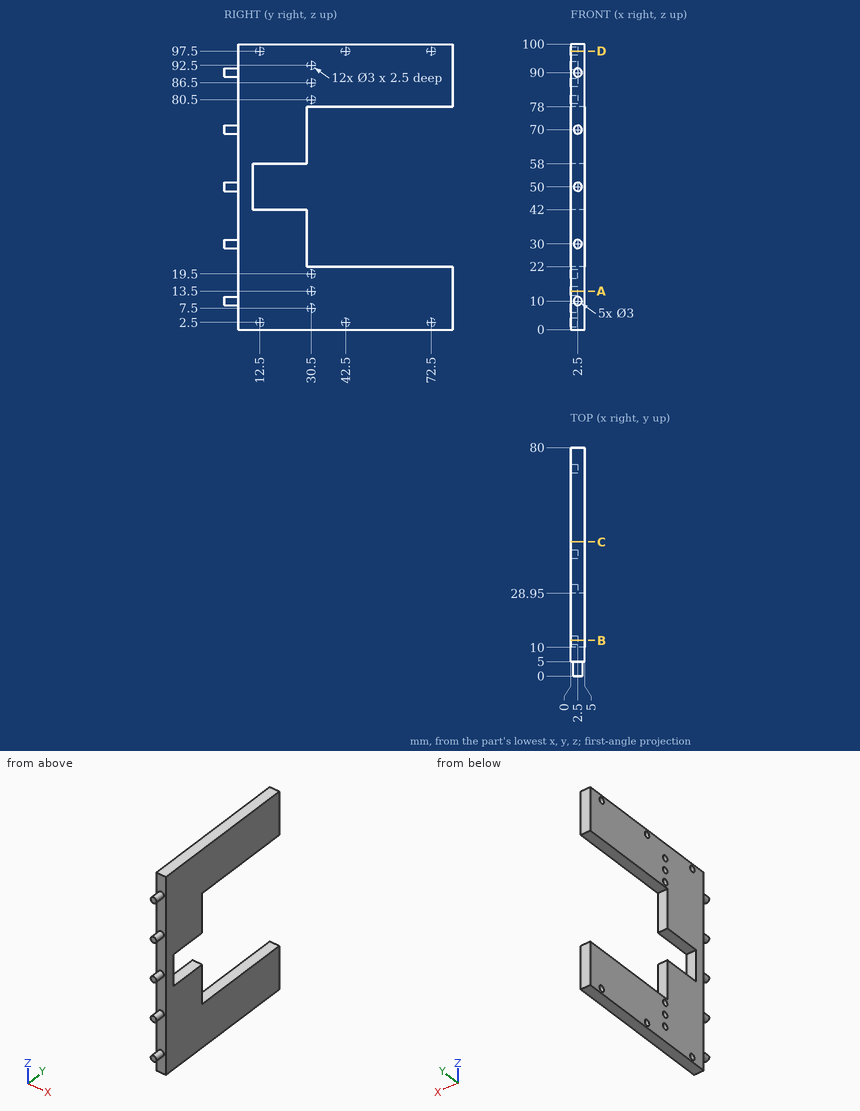
Geometry check sheet. Reference: drawing and pictorial views, mm from the part's lowest x, y, z. Coordinates: 2 decimals unless noted, no trailing zeros. Order: outer loops, then holes, each group sorted by start corner. A loop starts at its lowest first (then second) coordinate and runs counter-clockwise, first axis right, second up.
1. Scan lines: line 1 (Y direction, x = 1.1, z = 97.5); line 2 (Z direction, x = 2.4, y = 15); line 3 (Y direction, x = 0.6, z = 13.5). Record each from-to range of solid material in increasing order.
Results found:
line 1: y = 5 to 11, 14 to 41, 44 to 71, 74 to 80
line 2: z = 0 to 42, 58 to 100
line 3: y = 5 to 29, 32 to 80
2. Sectioned sample at A-A, the plane z = 13.5. Record the cut outline in (x, y).
Results found:
outline: (0, 5) - (5, 5) - (5, 80) - (0, 80) - (0, 32) - (2.5, 32) - (2.5, 29) - (0, 29) - close
3. Sectioned sample at D-D, the plane z = 97.5. Record the cut outline in (x, y).
Results found:
outline: (0, 5) - (5, 5) - (5, 80) - (0, 80) - (0, 74) - (2.5, 74) - (2.5, 71) - (0, 71) - (0, 44) - (2.5, 44) - (2.5, 41) - (0, 41) - (0, 14) - (2.5, 14) - (2.5, 11) - (0, 11) - close
4. Sectioned sample at C-C, the plane y = 47. Record the cut outline in (x, z), and give its area (3 significant figures).
Results found:
outline: (0, 0) - (5, 0) - (5, 22) - (0, 22) - close; (0, 78) - (5, 78) - (5, 100) - (0, 100) - close
area: 220 mm2
5. Go/stop test with flat-tipped pins: pin 1 Ø2 at (x, y) = (4.5, 60) entering from -Z; pin 2 Ø1.5 at (y, z) = (73, 2.5) entering from -X; pin 3 Ø2.5 at (x, z) = (3.5, 51) entering from +Y. Record where each tip stops, or that it passes through.
Results found:
pin 1: stops at z = 0
pin 2: stops at x = 2.5
pin 3: stops at y = 10
6. Sectioned sample at B-B, the plane y = 12.5. Record the cut outline in (x, z).
Results found:
outline: (0, 0) - (5, 0) - (5, 42) - (0, 42) - (0, 4) - (2.5, 4) - (2.5, 1) - (0, 1) - close; (0, 58) - (5, 58) - (5, 100) - (0, 100) - (0, 99) - (2.5, 99) - (2.5, 96) - (0, 96) - close
